Design review of the part built by this model. Coordinates are the model's own, in mm. Face numbers are marked on the shaded views. Round coordinates to 2 decimals unless told otherwise and drop trailing zeros. Loops run counter-clockwise (first coordinate to the right, second up) from the corner with the lowest first, then second, coordinate; pieces in that order, holes last. Notation, with made-up numbers: (-6, -6.5) - (25, -6.5) arc R28 ccw to (25, 26.5) - close; hole circle Ø10 at (3.5, -21.5). An arc over 180 degrees is marked (long way). Use one line per item in the form item = value. Start each with the question number.
(1) For pin 1 (1.5 mm diameter, centred on y = 27.5, z = 9, fed in from -X); pin 2 (3.5 mm diameter, centred on y = 1, z = 9, fed in from -X); pin 3 (3 mm diameter, centred on x = 24, y = 15, fed in from -Z); pin 4 (3.5 mm diameter, centred on x = 22.5, y = 13.5, fed in from +Z), all flat-tipped, find the tip position at first contact; note any pin that passes through.
(2) Wall thickness on probe 1 along X at (y, z) = (15, 0.9); probe 2 along Y at (x, z) = (24, 0.5); probe 3 along X at (y, z) = (1, 9.25): over which ranges is each line inside the solid? List them lowest first. Write a range as [from, to].
(3) We need section A-A, the plane x = 24. Write out the cut boundary in (y, z).
(4) We need section B-B, the plane y = 10. Write out the cut boundary in (x, z).
(5) The part is to be moulded in two halves that separate along X. For the marked faces 1, 2 and 3, say which applies: released by +X, released by -X, zero draft, split by the parting line, or undercut.
from build123d import *

# Parameters (mm, degrees)
SCHIZZO1_W                   = 155
SCHIZZO1_H                   = 70
ESTRUSIONE_ESTRUSIONE1_DEPTH = 6
ESTRUSIONE_ESTRUSIONE3_DEPTH = 5
ESTRUSIONE_ESTRUSIONE4_DEPTH = 20
SCHIZZO6_W                   = 8.5
SCHIZZO6_H                   = 70
ESTRUSIONE_ESTRUSIONE5_DEPTH = 6
SCHIZZO7_R                   = 1.75
TAGLIO_ESTRUSIONE2_DEPTH     = 94.498663092
FORO1_AT_2_COUNT             = 2
FORO1_AT_2_PITCH             = 100
SCHIZZO9_R                   = 3.5
TAGLIO_ESTRUSIONE3_DEPTH     = 94.112834821
SMUSSO1_SIZE                 = 2
TAGLIO_ESTRUSIONE4_DEPTH     = 30


with BuildPart() as part:
    # Schizzo1 → Estrusione-Estrusione1 (new body)
    with BuildSketch(Plane.XY):
        Rectangle(SCHIZZO1_W, SCHIZZO1_H)
    extrude(amount=ESTRUSIONE_ESTRUSIONE1_DEPTH)

    # Schizzo3 → Estrusione-Estrusione3 (add)
    with BuildSketch(Plane.XY.offset(6)):
        Polygon((-76, -33.5), (-76, 35), (-77.5, 35), (-77.5, -35), (-76, -35), align=None)
        Polygon((77.5, 35), (76, 35), (76, -33.5), (76, -35), (77.5, -35), align=None)
    extrude(amount=ESTRUSIONE_ESTRUSIONE3_DEPTH)

    # Schizzo4 → Estrusione-Estrusione4 (add)
    with BuildSketch(Plane(origin=(0, 35, 0), x_dir=(1, 0, 0), z_dir=(0, 1, 0))):
        with BuildLine():
            ThreePointArc((76, -8.5), (74.75, -9.75), (76, -11))
            Line((76, -11), (76, -8.5))
        make_face()
    estrusione_estrusione4 = extrude(amount=-ESTRUSIONE_ESTRUSIONE4_DEPTH)

    # Specchia1: Estrusione-Estrusione4 across plane
    add(estrusione_estrusione4.mirror(Plane(origin=(0, 0, 0), x_dir=(0, 0, 1), z_dir=(1, 0, 0))))

    # Schizzo6 → Estrusione-Estrusione5 (add)
    with BuildSketch(Plane.XY):
        with Locations((-81.75, 0)):
            Rectangle(SCHIZZO6_W, SCHIZZO6_H)
    extrude(amount=ESTRUSIONE_ESTRUSIONE5_DEPTH)

    # Schizzo7 → Taglio-Estrusione2 (cut, through all)
    with BuildSketch(Plane(origin=(0, 0, 0), x_dir=(-1, 0, 0), z_dir=(0, 0, -1))):
        with Locations((-24, 15)):
            Circle(SCHIZZO7_R)
        with Locations((76, 15)):
            Circle(SCHIZZO7_R)
    extrude(amount=-TAGLIO_ESTRUSIONE2_DEPTH, mode=Mode.SUBTRACT)

    # Schizzo8 → Foro1 (revolve, cut)
    with BuildSketch(Plane(origin=(24, 15, 6), x_dir=(0, -1, 0), z_dir=(1, 0, 0))):
        Polygon((0, 0), (0, 7.051506083), (1.75, 6), (1.75, 2), (3.5, 2), (3.5, 0), align=None)
    foro1 = revolve(axis=Axis((24, 15, 17.310875039), (0, 0, -1)), mode=Mode.SUBTRACT)

    # Foro1 at 2: Foro1 ×2
    with Locations(*[(-i * FORO1_AT_2_PITCH, 0, 0) for i in range(1, FORO1_AT_2_COUNT)]):
        add(foro1, mode=Mode.SUBTRACT)

    # Schizzo9 → Taglio-Estrusione3 (cut, through all)
    with BuildSketch(Plane.XY.offset(4)):
        with Locations((-76, 15)):
            Circle(SCHIZZO9_R)
    extrude(amount=TAGLIO_ESTRUSIONE3_DEPTH, mode=Mode.SUBTRACT)

    # Smusso1
    # the kernel refuses this chamfer: 2 mm, written as the material it adds along each edge
    with BuildSketch(Plane(origin=(-77.5, 13.018911684, 6), x_dir=(-0.9996219169112968, 0, -0.027495876610586414), z_dir=(0, 1, 0))) as smusso1_piece_1_section:
        Polygon((SMUSSO1_SIZE * 0.999621916911, SMUSSO1_SIZE * 0.0274958766106), (-SMUSSO1_SIZE * 0.0274958766106, SMUSSO1_SIZE * 0.999621916911), (0, 0), align=None)
    smusso1_piece_1 = extrude(amount=21.981088316, mode=Mode.PRIVATE)
    smusso1_piece_1 = smusso1_piece_1 - Plane(origin=(-76, 15, 6.650360418), x_dir=(0, -1, 0), z_dir=(0, 0, 1)) * Cylinder(3.5, 52, mode=Mode.PRIVATE)
    add(smusso1_piece_1)
    with BuildSketch(Plane(origin=(-77.5, -35, 6), x_dir=(0.02749587661058907, 0, 0.9996219169112965), z_dir=(0, 1, 0))) as smusso1_piece_2_section:
        Polygon((SMUSSO1_SIZE * 0.999621916911, -SMUSSO1_SIZE * 0.0274958766106), (-SMUSSO1_SIZE * 0.0274958766106, -SMUSSO1_SIZE * 0.999621916911), (0, 0), align=None)
    smusso1_piece_2 = extrude(amount=51.981088316, mode=Mode.PRIVATE)
    smusso1_piece_2 = smusso1_piece_2 - Plane(origin=(-76, 15, 6.656201353), x_dir=(1, 0, 0), z_dir=(0, 0, -1)) * Cylinder(3.5, 112, mode=Mode.PRIVATE)
    add(smusso1_piece_2)

    # Schizzo10 → Taglio-Estrusione4 (cut)
    with BuildSketch(Plane.XZ.offset(35)):
        Polygon((76, 11), (76, 6), (-76, 6), (-76, 11), (-77.5, 11), (-77.5, 8), (-79.5, 6), (-86, 6), (-86, 0), (77.5, 0), (77.5, 11), align=None)
    extrude(amount=-TAGLIO_ESTRUSIONE4_DEPTH, mode=Mode.SUBTRACT)


solid = part.part
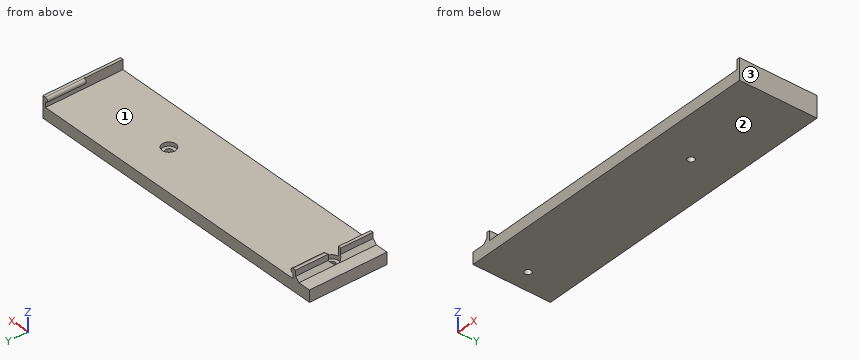
Data:
q1.pin_1 = -77.5
q1.pin_2 = -78.25
q1.pin_3 = through
q1.pin_4 = 6
q2.probe_1 = [-86, -77.75], [-74.25, 22.25], [25.75, 77.5]
q2.probe_2 = [-5, 13.25], [16.75, 35]
q2.probe_3 = [-77.5, -76], [76, 77.5]
q3.outline = (-5, 0) - (13.25, 0) - (13.25, 4) - (11.5, 4) - (11.5, 6) - (-5, 6) - close; (16.75, 0) - (35, 0) - (35, 6) - (18.5, 6) - (18.5, 4) - (16.75, 4) - close
q4.outline = (-86, 0) - (77.5, 0) - (77.5, 11) - (76, 11) - (76, 6) - (-76, 6) - (-76, 11) - (-77.5, 11) - (-77.5, 8) - (-79.5, 6) - (-86, 6) - close
q5.face_1 = undercut
q5.face_2 = zero draft
q5.face_3 = released by +X
